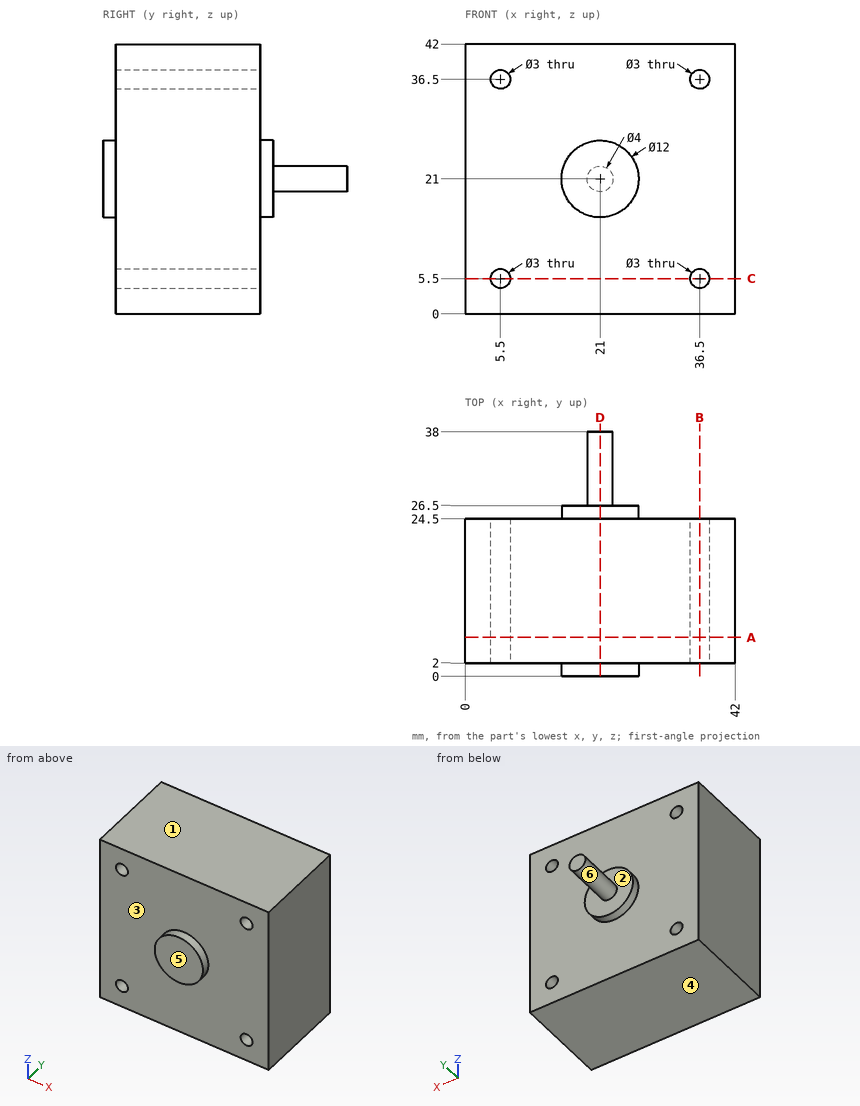
Check sheet for the drawn part. Datum: minimum x, y, z corner. Units: mm. A direction names the side the tool comes from. Round coordinates to 2 decimals unless told otherwise and drop trailing zeros. Order: outer loops, then holes, each group sorted by start corner. A loop starts at its lowest first (then second) coordinate and runs counter-clockwise, first axis right, second up. Notation, with made-up numbers: M -2.75,60.25 L 20.25,60.25 A22 ccw 20.25,99.25 Z; hole C -19.75,-24 d6. An arc over 180 degrees is marked long. Answer in a Markdown table with one row per item.
(1) Section check C-C on z = 5.5. Record the boundary of the cut face in (x, y), plus the area to 3 significant figures.
Findings:
| item | result |
|---|---|
| outline | M 0,2 L 4,2 L 4,24.5 L 0,24.5 Z; M 7,2 L 35,2 L 35,24.5 L 7,24.5 Z; M 38,2 L 42,2 L 42,24.5 L 38,24.5 Z |
| area | 810 mm^2 |
(2) Material ranges on line 1 along Z through (x, y) = (5.5, 10.5); line 2 along X through (y, z) = (11, 36), recorded low to high. Write a range as from..to.
Findings:
| item | result |
|---|---|
| line 1 | z = 0..4, 7..35, 38..42 |
| line 2 | x = 0..4.09, 6.91..35.09, 37.91..42 |
(3) Section check B-B on x = 36.5. Record the boundary of the cut face in (y, z), plus the area to 3 significant figures.
Findings:
| item | result |
|---|---|
| outline | M 2,0 L 24.5,0 L 24.5,4 L 2,4 Z; M 2,7 L 24.5,7 L 24.5,35 L 2,35 Z; M 2,38 L 24.5,38 L 24.5,42 L 2,42 Z |
| area | 810 mm^2 |
(4) Draft check along Z on the marked faces 4, 5 and 6. Enter one of: +Z half, -Z half, draft (parallel to the pull), parting line (faces both ways), or undercut.
Findings:
| item | result |
|---|---|
| face 4 | -Z half |
| face 5 | draft |
| face 6 | parting line |
(5) Section check A-A on y = 6. Record the boundary of the cut face in (x, z).
Findings:
| item | result |
|---|---|
| outline | M 0,0 L 42,0 L 42,42 L 0,42 Z; hole C 5.5,5.5 d3; hole C 5.5,36.5 d3; hole C 36.5,5.5 d3; hole C 36.5,36.5 d3 |
(6) Set-up check for the marked faces 1, 2 and 3: record each of +Z, -Z, +X, -X, +Y, -Y from which the full face is reachable in a straight line by a thin tool's end or side.
Findings:
| item | result |
|---|---|
| face 1 | +Z, +X, -X, +Y, -Y |
| face 2 | +Y |
| face 3 | -Y |
(7) Gauge pin test, flat ends, axial feed: pin 1 (2 mm diameter, centred on x = 11.5, z = 9, fed in from +Y); pin 2 (5 mm diameter, centred on x = 18.5, y = 31, fed in from -Z); pin 3 (12.5 mm diameter, centred on x = 29, z = 24.5, fed in from +Y). Record the tip position at first contact, or that the pin passes through.
Findings:
| item | result |
|---|---|
| pin 1 | stops at y = 24.5 |
| pin 2 | stops at z = 19 |
| pin 3 | stops at y = 26.5 |
(8) Section check D-D on x = 21. Record the boundary of the cut face in (y, z), plus the area to 3 significant figures.
Findings:
| item | result |
|---|---|
| outline | M 0,15 L 2,15 L 2,0 L 24.5,0 L 24.5,15 L 26.5,15 L 26.5,19 L 38,19 L 38,23 L 26.5,23 L 26.5,27 L 24.5,27 L 24.5,42 L 2,42 L 2,27 L 0,27 Z |
| area | 1,040 mm^2 |
